Check sheet for the modelled part. Datum: model origin and axes. Units: mm. Give positions to 0.01 mm unless a question says otherwise; leave off trailing zeros. Loops run counter-clockwise (first coordinate to the right, second up) from the corner with the lowest first, then second, coordinate; pieces in that order, holes last. Notation, with made-up numbers: (18, 62.25) - (68, 62.25) arc R7 cw to (68, 68.25) - close; hole circle Ø8 at (10, 65.5). An arc over 180 degrees is marked (long way). Use one line per item in the form item = value.
from build123d import *

# Parameters (mm, degrees)
F0_R          = 5
F0_W          = 2.5
F0_H          = 2.5
F1_DEPTH      = 25
F2_DEPTH      = 4
F3_R          = 1
F5_DEPTH      = 25
F5_DEPTH_BACK = 25


with BuildPart() as f1:
    # F0 (on Top) → F1 (new body)
    with BuildSketch(Plane.XY):
        Circle(F0_R)
        Rectangle(F0_W, F0_H, mode=Mode.SUBTRACT)
    extrude(amount=F1_DEPTH)

    # F0 (on Top) → F2 (join)
    with BuildSketch(Plane.XY):
        Rectangle(F0_W, F0_H)
    extrude(amount=F2_DEPTH)

    # F3
    f3_edges = [f1.edges().sort_by_distance(p)[0] for p in [
        (-5, 0, 0),
    ]]
    fillet(f3_edges, radius=F3_R)

    # F4 (on Front) → F5 (cut, two sides)
    with BuildSketch(Plane.XZ) as f5_sk:
        Polygon((-9.264733, 30.193007), (-9.264733, 15.788589), (12.869327, 28.567694), (-3.567463, 35.245303), align=None)
    extrude(amount=F5_DEPTH, mode=Mode.SUBTRACT)
    extrude(f5_sk.sketch, amount=-F5_DEPTH_BACK, mode=Mode.SUBTRACT)


solid = f1.part
Item 1: Mould release check, pull along X, two halves, no side actions. Record for faces 1 (the face through (4.77, 1.5, 12.35)), 2 (the face through (0, 1.25, 13)), 3 (the face through (0, 0, 0)), 4 (the face through (-0.07, -2.152, 21.097)): released by +X, released by -X, zero draft, split by the parting line, or undercut.
Answer block:
face_1 = split by the parting line
face_2 = undercut
face_3 = zero draft
face_4 = released by -X
Item 2: Thickness scan on L1, parallel to X at y = 0.25, z = 18; L2, parallel to Y at x = 0, z = 10; L3, parallel to Z at x = -0.25, y = -0.5. Record the ranges inside material, lowest first.
Answer block:
L1 = -4.99 to -1.25, 1.25 to 4.99
L2 = -5 to -1.25, 1.25 to 5
L3 = 0 to 4
Item 3: Section check C-C on x = 0. Record the boundary of the cut face in (y, z).
Answer block:
outline = (-5, 1) arc R1 ccw to (-4, 0) - (4, 0) arc R1 ccw to (5, 1) - (5, 21.14) - (1.25, 21.14) - (1.25, 4) - (-1.25, 4) - (-1.25, 21.14) - (-5, 21.14) - close
Item 4: Section check A-A on z = 18. Record the boundary of the cut face in (x, y).
Answer block:
outline = circle Ø10 at (0, 0); hole (-1.25, -1.25) - (1.25, -1.25) - (1.25, 1.25) - (-1.25, 1.25) - close
Item 5: Section check B-B on y = 0. Record the boundary of the cut face in (x, z).
Answer block:
outline = (-5, 1) arc R1 ccw to (-4, 0) - (4, 0) arc R1 ccw to (5, 1) - (5, 24.02) - (1.25, 21.86) - (1.25, 4) - (-1.25, 4) - (-1.25, 20.42) - (-5, 18.25) - close
Item 6: Gauge pin test, flat ends, axial feed: P1, Ø6, axis at x = 3, z = 2.5, coming from the -Y side; P2, Ø1.5, axis at y = 1.5, z = 12.5, coming from the -X side; P3, Ø2, axis at x = -0.5, y = 0.5, coming from the +Z side. Record the tip position at first contact, or that the pin passes through.
Answer block:
P1 = -5
P2 = -4.94
P3 = 21.23
